Could you check a few things on this model? Use its own coordinates, in mm. A direction names the side the tool comes from. Give positions to 0.01 mm unless a question says otherwise; leave off trailing zeros. Write each loop counter-clockwise with the first axis right and the second up, starting at its lowest first coordinate (ties: lowest second). Pieces come first, ordered by that corner, then holes. Notation, with made-up numbers: (0, 78) - (22, 78) arc R13 ccw to (22, 103) - close; hole circle Ø2 at (89, -2). An arc over 180 degrees is marked (long way). Answer in a Markdown table with one row per item.
from build123d import *

# Parameters (mm, degrees)
F1_DEPTH = 50.8
F2_SIZE  = 5.08
F4_DEPTH = 12.7
F5_R     = 5.08
F6_R     = 5.08


with BuildPart() as f1:
    # F0 (on Top) → F1 (new body)
    with BuildSketch(Plane.XY):
        with BuildLine():
            ThreePointArc((11.4679807678, -33.227154294), (28.6239736934, -20.4016297233), (35.1505101722, 0))
            ThreePointArc((35.1505101722, 0), (27.5943099323, 21.7741228234), (8.1743768298, 34.186809281))
            Line((8.1743768298, 34.186809281), (8.1743768298, 17.2070352892))
            ThreePointArc((8.1743768298, 17.2070352892), (16.1031732681, 10.1779325354), (19.05, 0))
            ThreePointArc((19.05, 0), (16.1031732681, -10.1779325354), (8.1743768298, -17.2070352892))
            Line((8.1743768298, -17.2070352892), (8.1743768298, -33.227154294))
            Line((8.1743768298, -33.227154294), (11.4679807678, -33.227154294))
        make_face()
        with BuildLine():
            ThreePointArc((8.1743768298, 34.186809281), (27.5943099323, 21.7741228234), (35.1505101722, 0))
            ThreePointArc((35.1505101722, 0), (28.6239736934, -20.4016297233), (11.4679807678, -33.227154294))
            Line((11.4679807678, -33.227154294), (60.3725549432, -33.227154294))
            Line((60.3725549432, -33.227154294), (60.3725549432, 34.186809281))
            Line((60.3725549432, 34.186809281), (8.1743768298, 34.186809281))
        make_face()
        with BuildLine():
            Line((8.1743768298, 17.2070352892), (8.1743768298, 34.186809281))
            ThreePointArc((8.1743768298, 34.186809281), (-35.1086338985, -1.7152816528), (11.4679807678, -33.227154294))
            Line((11.4679807678, -33.227154294), (8.1743768298, -33.227154294))
            Line((8.1743768298, -33.227154294), (8.1743768298, -17.2070352892))
            ThreePointArc((8.1743768298, -17.2070352892), (-19.05, 0), (8.1743768298, 17.2070352892))
        make_face()
    extrude(amount=F1_DEPTH)

    # F2
    f2_edges = [f1.edges().sort_by_distance(p)[0] for p in [
        (-35.108634, -1.715282, 0),
        (34.273466, 34.186809, 0),
        (60.372555, 0.479827, 0),
        (35.920268, -33.227154, 0),
    ]]
    chamfer(f2_edges, length=F2_SIZE)

    # F3 (on Top) → F4 (join)
    with BuildSketch(Plane.XY):
        with BuildLine():
            Line((9.958841659, 26.0848395173), (9.958841659, -26.0848395173))
            ThreePointArc((9.958841659, -26.0848395173), (22.9963138093, -15.8356222175), (27.9212710998, 0))
            ThreePointArc((27.9212710998, 0), (22.9963138093, 15.8356222175), (9.958841659, 26.0848395173))
        make_face()
        with BuildLine():
            ThreePointArc((27.9212710998, 0), (22.9963138093, -15.8356222175), (9.958841659, -26.0848395173))
            Line((9.958841659, -26.0848395173), (51.6148433089, -26.0848395173))
            Line((51.6148433089, -26.0848395173), (51.6148433089, 26.8565043807))
            Line((51.6148433089, 26.8565043807), (9.958841659, 26.8565043807))
            Line((9.958841659, 26.8565043807), (9.958841659, 26.0848395173))
            ThreePointArc((9.958841659, 26.0848395173), (22.9963138093, 15.8356222175), (27.9212710998, 0))
        make_face()
        with BuildLine():
            ThreePointArc((9.958841659, 26.0848395173), (-27.9212710998, 0), (9.958841659, -26.0848395173))
            Line((9.958841659, -26.0848395173), (9.958841659, 26.0848395173))
        make_face()
    extrude(amount=F4_DEPTH)

    # F5
    f5_edges = [f1.edges().sort_by_distance(p)[0] for p in [
        (-35.108634, -1.715282, 50.8),
        (35.920268, -33.227154, 50.8),
        (60.372555, 0.479827, 50.8),
        (34.273466, 34.186809, 50.8),
    ]]
    fillet(f5_edges, radius=F5_R)

    # F6
    f6_edges = [f1.edges().sort_by_distance(p)[0] for p in [
        (-8.174377, 17.207035, 50.8),
    ]]
    fillet(f6_edges, radius=F6_R)


solid = f1.part
1) We'd pull the mould along X, two halves only. Please class faces 1 (the face through (-35.14, -0.8, 25.12)), 2 (the face through (36, -33.227, 25)), 3 (the face through (60.373, 0, 25)), 4 (the face through (0, 0, 12.7)): +X half, -X half, draft (parallel to the pull), parting line (faces both ways), or undercut.
Check values:
| item | result |
|---|---|
| face 1 | parting line |
| face 2 | draft |
| face 3 | +X half |
| face 4 | undercut |
2) Imagine slicing it at A-A (z = 23.5). List the corners of the cut face in (x, y) for me, then the cut area to 3 significant figures.
Check values:
| item | result |
|---|---|
| outline | (8.17, 34.19) arc R35.15 ccw (long way) to (11.47, -33.23) - (60.37, -33.23) - (60.37, 34.19) - close; hole circle Ø38.1 at (0, 0) |
| area | 4,890 mm2 |
3) On a 3-axis mill with a long thin cutter (end or side, diameter ignored), from which of +Z, -Z, +X, -X, +Y, -Y can I reach the whole of each face in a straight line? I mean faces 5 (the face through (35.129, -30.652, 2.504)), 6 (the face through (35.83, -31.78, 49.27)), 7 (the face through (33.59, 32.74, 49.27)), 8 (the face through (34.332, 31.611, 2.504)). Say none if no direction works.
Check values:
| item | result |
|---|---|
| face 5 | -Z, +X, -Y |
| face 6 | +Z, +X, -Y |
| face 7 | +Z, +X, +Y |
| face 8 | -Z, +X, +Y |
4) Imagine slicing it at B-B (x = 48.5). List the corners of the cut face in (y, z) for me, then the cut area to 3 significant figures.
Check values:
| item | result |
|---|---|
| outline | (-33.23, 5.08) - (-28.15, 0) - (29.11, 0) - (34.19, 5.08) - (34.19, 45.72) arc R5.08 ccw to (29.11, 50.8) - (-28.15, 50.8) arc R5.08 ccw to (-33.23, 45.72) - close |
| area | 3,390 mm2 |
5) Will these pins go through, and if not, where does the flat tip stop? P1, Ø12, axis at x = 36, z = 31.5, coming from the -Y side; P2, Ø12, axis at x = -11, y = -4, coming from the +Z side; P3, Ø10, axis at y = 22, z = 28.5, coming from the -X side.
Check values:
| item | result |
|---|---|
| P1 | stops at y = -33.23 |
| P2 | stops at z = 12.7 |
| P3 | stops at x = -30.77 |
6) If I drill on line 1 (Y direction, x = 0, z = 38); line 2 (Y direction, x = 34.5, z = 23); line 3 (Z direction, x = -22.5, y = -8), over which ranges is the centre line in solid material (lowest first)?
Check values:
| item | result |
|---|---|
| line 1 | y = -35.15 to -19.05, 19.05 to 35.15 |
| line 2 | y = -33.23 to 34.19 |
| line 3 | z = 0 to 50.79 |
